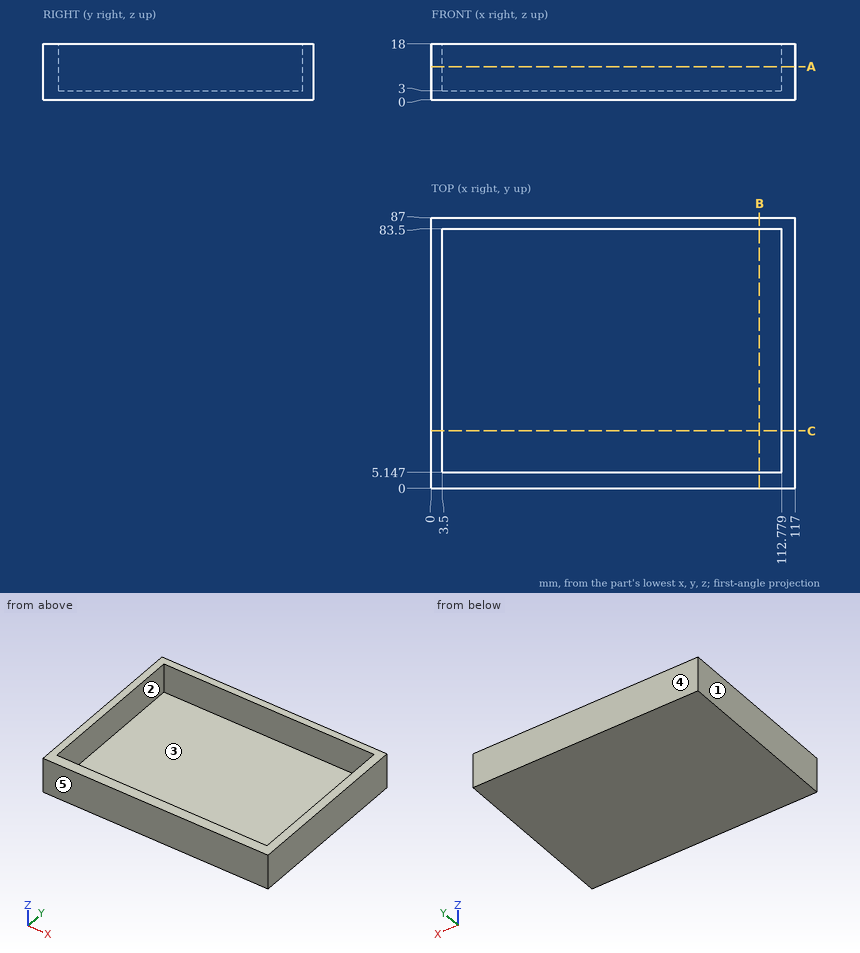
Source: three-view drawing plus pictorial views. Frame: mm from the lowest corner of the part. A direction names the side the tool comes from. Coordinates: 2 decimals unless noted, no trailing zeros. Write each loop counter-clockwise with the first axis right and the second up, starting at its lowest first coordinate (ties: lowest second). Pieces come first, ordered by that corner, then holes. Notation, with made-up numbers: (50, 56) - (81, 56) arc R15 ccw to (81, 80) - close; hole circle Ø7 at (-28.5, 55.5). An arc over 180 degrees is marked (long way). Answer as a JSON object with one key per item and string values.
Q1. Set-up query: the marked faces 1 and 2. Return all of +Z, -Z, +X, -X, +Y, -Y with unobstructed straight access to the full face (end or side cutting, diameter ignored); none if empty.
Ans:
{"face 1": "+Z, -Z, -X, +Y, -Y", "face 2": "+Z"}
Q2. First-contact query: pin 1 Ø4.5 at (x, z) = (35.5, 13) entering from -Y; pin 2 Ø1 at (x, y) = (37, 71.5) entering from +Z. Flat tips, straight axial feed; report the tip coordinate or a pass-through.
Ans:
{"pin 1": "stops at y = 0", "pin 2": "stops at z = 3"}
Q3. Section query C-C, the plane y = 18.5. Output: boundary loops of the cut face in (x, z).
Ans:
{"outline": "(0, 0) - (117, 0) - (117, 18) - (112.78, 18) - (112.78, 3) - (3.5, 3) - (3.5, 18) - (0, 18) - close"}
Q4. Section query B-B, the plane x = 105.5. Output: boundary loops of the cut face in (y, z).
Ans:
{"outline": "(0, 0) - (87, 0) - (87, 18) - (83.5, 18) - (83.5, 3) - (5.15, 3) - (5.15, 18) - (0, 18) - close"}
Q5. Section query A-A, the plane z = 10.75. Output: boundary loops of the cut face in (x, y).
Ans:
{"outline": "(0, 0) - (117, 0) - (117, 87) - (0, 87) - close; hole (3.5, 5.15) - (112.78, 5.15) - (112.78, 83.5) - (3.5, 83.5) - close"}
Q6. Draft query along Y for the marked faces 3, 4 and 5. Return one class per face: released by +Y, released by -Y, zero draft, split by the parting line, or undercut.
Ans:
{"face 3": "undercut", "face 4": "released by +Y", "face 5": "released by -Y"}
Q7. Material intervals for line 1 (X direction, y = 21.5, z = 14.5); line 2 (Y direction, x = 64.5, z = 14.5); line 3 (Z direction, x = 17.5, y = 71), sorted ascending. Write a range as [from, to].
Ans:
{"line 1": "x = [0, 3.5], [112.78, 117]", "line 2": "y = [0, 5.15], [83.5, 87]", "line 3": "z = [0, 3]"}
